```python
from build123d import *

# Parameters (mm, degrees)
BOSS_EXTRUDE1_DEPTH     = 30
SKETCH3_4_R             = 10
BOSS_EXTRUDE2_DEPTH     = 10
SKETCH4_R               = 1.5
SKETCH4_R_2             = 2
CUT_EXTRUDE1_DEPTH      = 10
CUT_EXTRUDE2_DEPTH      = 28
CUT_EXTRUDE2_DEPTH_BACK = 28
SKETCH6_W               = 22
SKETCH6_H               = 41
SKETCH6_R               = 10
CUT_EXTRUDE3_DEPTH      = 8
SKETCH6_3_R             = 1.5
CUT_EXTRUDE4_DEPTH      = 11.0000001
CUT_EXTRUDE5_DEPTH      = 68.0000001


with BuildPart() as part:
    # Sketch3 → Boss-Extrude1 (new body)
    with BuildSketch(Plane.XY):
        with BuildLine():
            ThreePointArc((-27, 20), (0, 47), (27, 20))
            Line((27, 20), (27, -20))
            Line((27, -20), (-27, -20))
            Line((-27, -20), (-27, 20))
        make_face()
        with BuildLine():
            Line((-24, -17), (-24, 20))
            ThreePointArc((-24, 20), (0, 44), (24, 20))
            Line((24, 20), (24, -17))
            Line((24, -17), (-24, -17))
        make_face(mode=Mode.SUBTRACT)
    extrude(amount=-BOSS_EXTRUDE1_DEPTH)

    # Sketch3<4> → Boss-Extrude2 (add)
    with BuildSketch(Plane.XY):
        with BuildLine():
            ThreePointArc((-24, 20), (0, 44), (24, 20))
            Line((24, 20), (24, -17))
            Line((24, -17), (-24, -17))
            Line((-24, -17), (-24, 20))
        make_face()
        with Locations((0, 20)):
            Circle(SKETCH3_4_R, mode=Mode.SUBTRACT)
    extrude(amount=-BOSS_EXTRUDE2_DEPTH)

    # Sketch4 → Cut-Extrude1 (cut)
    with BuildSketch(Plane.XZ.offset(20)):
        with Locations((3, -15)):
            Circle(SKETCH4_R)
        with Locations((17, -15)):
            Circle(SKETCH4_R)
        with Locations((10, -15)):
            Circle(SKETCH4_R_2)
    extrude(amount=-CUT_EXTRUDE1_DEPTH, mode=Mode.SUBTRACT)

    # Sketch5 → Cut-Extrude2 (cut, two sides)
    with BuildSketch(Plane(origin=(0, 0, 0), x_dir=(0, 0, -1), z_dir=(1, 0, 0))) as cut_extrude2_sk:
        with BuildLine():
            Line((15.255034443, 32.183889783), (30, -15))
            Line((30, -15), (30, 47))
            Line((30, 47), (15, 47))
            ThreePointArc((15, 47), (14.181044165, 40.740478791), (14.690093427, 34.448168938))
            ThreePointArc((14.690093427, 34.448168938), (14.93950997, 33.307782347), (15.255034443, 32.183889783))
        make_face()
    extrude(amount=CUT_EXTRUDE2_DEPTH, mode=Mode.SUBTRACT)
    extrude(cut_extrude2_sk.sketch, amount=-CUT_EXTRUDE2_DEPTH_BACK, mode=Mode.SUBTRACT)

    # Sketch6 → Cut-Extrude3 (cut)
    with BuildSketch(Plane(origin=(0, 0, -10), x_dir=(-1, 0, 0), z_dir=(0, 0, -1))):
        with Locations((0, 10.5)):
            Rectangle(SKETCH6_W, SKETCH6_H)
        with Locations((0, 20)):
            Circle(SKETCH6_R, mode=Mode.SUBTRACT)
    extrude(amount=-CUT_EXTRUDE3_DEPTH, mode=Mode.SUBTRACT)

    # Sketch6<3> → Cut-Extrude4 (cut, through all)
    with BuildSketch(Plane(origin=(0, 0, -10), x_dir=(-1, 0, 0), z_dir=(0, 0, -1))):
        with Locations((-5, 34.5)):
            Circle(SKETCH6_3_R)
        with Locations((5, 34.5)):
            Circle(SKETCH6_3_R)
        with Locations((5, -13.5)):
            Circle(SKETCH6_3_R)
        with Locations((-5, -13.5)):
            Circle(SKETCH6_3_R)
    extrude(amount=-CUT_EXTRUDE4_DEPTH, mode=Mode.SUBTRACT)

    # Sketch7 → Cut-Extrude5 (cut, through all)
    with BuildSketch(Plane.XZ.offset(20)):
        with BuildLine():
            Line((-27, -25), (-27, -30))
            Line((-27, -30), (-22, -30))
            ThreePointArc((-22, -30), (-25.535533906, -28.535533906), (-27, -25))
        make_face()
        with BuildLine():
            Line((22, -30), (27, -30))
            Line((27, -30), (27, -25))
            ThreePointArc((27, -25), (25.535533906, -28.535533906), (22, -30))
        make_face()
    extrude(amount=-CUT_EXTRUDE5_DEPTH, mode=Mode.SUBTRACT)


solid = part.part
```
For this review, take the finished solid that the model builds, in its own axes (mm). A direction names the side the tool comes from. Give positions to 0.01 mm unless a question says otherwise; leave off trailing zeros. Order: outer loops, then holes, each group sorted by start corner. A loop starts at its lowest first (then second) coordinate and runs counter-clockwise, first axis right, second up.
1) Take a section at A-A (y = 15.5). Give the boundary of the cut face in (x, z), then the cut area to 3 significant figures.
2) Wall thickness on line 1 (Z direction, x = 3, y = -18.75); line 2 (Z direction, x = 10, y = -19); line 3 (X direction, y = -5.5, z = -18.5): over which ranges is each line inside the solid? List them lowest first.
3) Take a section at D-D (x = 17). Give the boundary of the cut face in (y, z).
4) Take a section at C-C (x = 2.5). Give the boundary of the cut face in (y, z).
5) Insertion check: pin 1 (8 mm diameter, centred on x = 12.5, z = -13, fed in from +Y); pin 2 (6.5 mm diameter, centred on x = 3.5, y = 11.5, fed in from -Z); pin 3 (1.5 mm diameter, centred on y = 29, z = -3.5, fed in from -X). Each pin has a flat end and moves straight along its axis. Give the tip position at first contact, or say it passes through.
6) For faces 4 (the face through (24, -2, -17)), 5 (the face through (-5, 33, -5)), list the 3-axis set-ups (+Z, -Z, +X, -X, +Y, -Y) from which the entire face can be reached by the end or side of a thin tool; tool diameter is ignored.
7) The part is to be moulded in two halves that separate along Z. For faces 1 (the face through (-26, -14, -28)), 2 (the face through (4.386, -18.521, -15.575)), 3 (the face through (-6.386, -14.075, -5.07)), say which applies: released by +Z, released by -Z, zero draft, split by the parting line, or undercut.
8) Take a section at B-B (x = -5). Give the boundary of the cut face in (y, z), then the cut area to 3 significant figures.
Derived:
1. outline: (-27, -20.47) - (-24, -20.47) - (-24, -10) - (-11, -10) - (-11, -2) - (-8.93, -2) - (-8.93, 0) - (-27, 0) - close; (8.93, -2) - (11, -2) - (11, -10) - (24, -10) - (24, -20.47) - (27, -20.47) - (27, 0) - (8.93, 0) - close
1. area: 391 mm2
2. line 1: z = -30 to -16.5, -13.5 to 0
2. line 2: z = -30 to -17, -13 to 0
2. line 3: x = -27 to -24, 24 to 27
3. outline: (-20, -30) - (-17, -30) - (-17, -16.5) - (-20, -16.5) - close; (-20, -13.5) - (-17, -13.5) - (-17, -10) - (36.94, -10) - (36.94, -14.33) arc R30 cw to (40.98, -14.19) - (40.98, 0) - (-20, 0) - close
4. outline: (-20, -30) - (-17, -30) - (-17, -16.41) - (-20, -16.41) - close; (-20, -13.59) - (-17, -13.59) - (-17, -10) - (-10, -10) - (-10, -2) - (10.32, -2) - (10.32, 0) - (-20, 0) - close; (29.68, -2) - (31, -2) - (31, -10) - (43.87, -10) - (43.87, -14.42) arc R30 cw to (46.88, -14.97) - (46.88, 0) - (29.68, 0) - close
5. pin 1: stops at y = 45.63
5. pin 2: stops at z = -2
5. pin 3: stops at x = -25.71
6. face 4: -Z
6. face 5: +Z, -Z
7. face 1: released by -Z
7. face 2: undercut
7. face 3: zero draft
8. outline: (-20, -30) - (-17, -30) - (-17, -10) - (-15, -10) - (-15, 0) - (-20, 0) - close; (-12, -10) - (-10, -10) - (-10, -2) - (11.34, -2) - (11.34, 0) - (-12, 0) - close; (28.66, -2) - (31, -2) - (31, -10) - (33, -10) - (33, 0) - (28.66, 0) - close; (36, -10) - (43.47, -10) - (43.47, -14.37) arc R30 cw to (46.53, -14.89) - (46.53, 0) - (36, 0) - close
8. area: 317 mm2
